Design review of the part built by this model. Coordinates are the model's own, in mm. Face numbers are marked on the shaded views. Coordinates: 2 decimals unless noted, no trailing zeros. Loops run counter-clockwise (first coordinate to the right, second up) from the corner with the lowest first, then second, coordinate; pieces in that order, holes last.
Q1. Add section A-A on y = 22.5. Give the boundary of the cut face in (x, z).
Q2. Draft analysis for pull direction X (two halves, no side actions). For the marked faces 1, 2 and 3, state which applies: released by +X, released by -X, zero draft, split by the parting line, or undercut.
Q3. Wall thickness on probe 1 along Y at (x, z) = (-13, 5); probe 2 along Y at (x, z) = (-9, -2.5); probe 3 along X at (y, z) = (20.5, -7.5): over which ranges is each line inside the solid? List them lowest first.
Q4. Add section B-B on z = 0.25. Give the boundary of the cut face in (x, y), and give its area (3 significant figures).
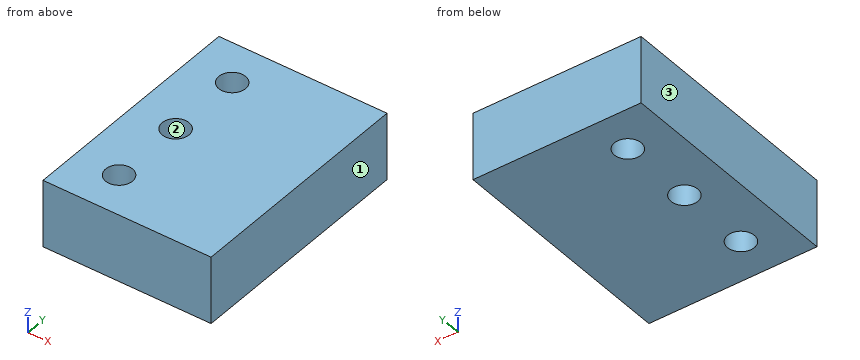
```python
from build123d import *

# Parameters (mm, degrees)
SKETCH1_W           = 50
SKETCH1_H           = 70
SKETCH1_R           = 4
BOSS_EXTRUDE1_DEPTH = 10


with BuildPart() as part:
    # Sketch1 → Boss-Extrude1 (new body, symmetric)
    with BuildSketch(Plane.XY):
        Rectangle(SKETCH1_W, SKETCH1_H)
        with Locations((-11.712149785, 0)):
            Circle(SKETCH1_R, mode=Mode.SUBTRACT)
        with Locations((-11.712149785, 22.5)):
            Circle(SKETCH1_R, mode=Mode.SUBTRACT)
        with Locations((-11.712149785, -22.5)):
            Circle(SKETCH1_R, mode=Mode.SUBTRACT)
    extrude(amount=BOSS_EXTRUDE1_DEPTH, both=True)


solid = part.part
```
Entries:
1. outline: (-25, -10) - (-15.71, -10) - (-15.71, 10) - (-25, 10) - close; (-7.71, -10) - (25, -10) - (25, 10) - (-7.71, 10) - close
2. face 1: released by +X
2. face 2: undercut
2. face 3: released by -X
3. probe 1: y = -35 to -26.29, -18.71 to -3.79, 3.79 to 18.71, 26.29 to 35
3. probe 2: y = -35 to -25.44, -19.56 to -2.94, 2.94 to 19.56, 25.44 to 35
3. probe 3: x = -25 to -15.18, -8.25 to 25
4. outline: (-25, -35) - (25, -35) - (25, 35) - (-25, 35) - close; hole circle Ø8 at (-11.71, -22.5); hole circle Ø8 at (-11.71, 0); hole circle Ø8 at (-11.71, 22.5)
4. area: 3,350 mm2
